Read the model definition and answer for the solid it produces. Units are mm, in the model's axes. A direction names the side the tool comes from. Coordinates: 2 decimals unless noted, no trailing zeros. Loops run counter-clockwise (first coordinate to the right, second up) from the corner with the lowest first, then second, coordinate; pieces in that order, holes last. Notation, with made-up numbers: (15.25, 84.25) - (64.25, 84.25) arc R7 cw to (64.25, 88.25) - close; hole circle Ø8 at (55, 66). An arc over 180 degrees is marked (long way). Use one line per item in the form item = value.
from build123d import *

# Parameters (mm, degrees)
SKETCH_5_W      = 32
SKETCH_5_H      = 28
EXTRUDE_5_DEPTH = 10
EXTRUDE_6_DEPTH = 9
CHAMFER_4_SIZE  = 0.5


with BuildPart() as part:
    # 草图5 → 凸台-拉伸5 (new body)
    with BuildSketch(Plane.XY):
        Rectangle(SKETCH_5_W, SKETCH_5_H)
    extrude(amount=EXTRUDE_5_DEPTH)

    # 草图6 → 凸台-拉伸6 (add)
    with BuildSketch(Plane.XY.offset(10)):
        Polygon((0, 14), (6.5, 14), (6.5, -14), (-6.5, -14), (-6.5, 14), align=None)
    extrude(amount=EXTRUDE_6_DEPTH)

    # 倒角4
    chamfer_4_edges = [part.edges().sort_by_distance(p)[0] for p in [
        (0, 14, 19),
        (-6.5, 0, 19),
        (0, -14, 19),
        (6.5, 0, 19),
    ]]
    chamfer(chamfer_4_edges, length=CHAMFER_4_SIZE)


solid = part.part
Item 1: The part is cut by section A-A on y = 8. Give the vertices of the cut face in (x, z).
Results below:
outline = (-16, 0) - (16, 0) - (16, 10) - (6.5, 10) - (6.5, 18.5) - (6, 19) - (-6, 19) - (-6.5, 18.5) - (-6.5, 10) - (-16, 10) - close
Item 2: The part is cut by section B-B on z = 17. Give the vertices of the cut face in (x, y).
Results below:
outline = (-6.5, -14) - (6.5, -14) - (6.5, 14) - (-6.5, 14) - close
Item 3: Each of these flat-tipped pins is pushed along its axis until it touches: P1, Ø3, axis at x = 13, y = 5, coming from the +Z side; P2, Ø2.5, axis at y = 6, z = 14.5, coming from the +X side; P3, Ø2.5, axis at y = 3, z = 15, coming from the -X side. Where does it stop, or does it pass through?
Results below:
P1 = 10
P2 = 6.5
P3 = -6.5
Item 4: Which of the six approach directions +Z, -Z, +X, -X, +Y, -Y give full straight-line access (tool end or side, diameter ignored) to faces 1 (the flat face through (-6.5, 0, 14)), 2 (the flat face through (6.5, 0, 14)), 3 (the flat face through (0, 0, 19))?
Results below:
face_1 = +Z, -X, +Y, -Y
face_2 = +Z, +X, +Y, -Y
face_3 = +Z, +X, -X, +Y, -Y
Item 5: The part is cut by section C-C on x = 8.5. Give the vertices of the cut face in (y, z).
Results below:
outline = (-14, 0) - (14, 0) - (14, 10) - (-14, 10) - close
Item 6: Find the intervals of material crossed by L1, parallel to X at y = 0.75, z = 15.25; L2, parallel to Z at x = 15, y = 8.5, in increasing order.
Results below:
L1 = -6.5 to 6.5
L2 = 0 to 10
